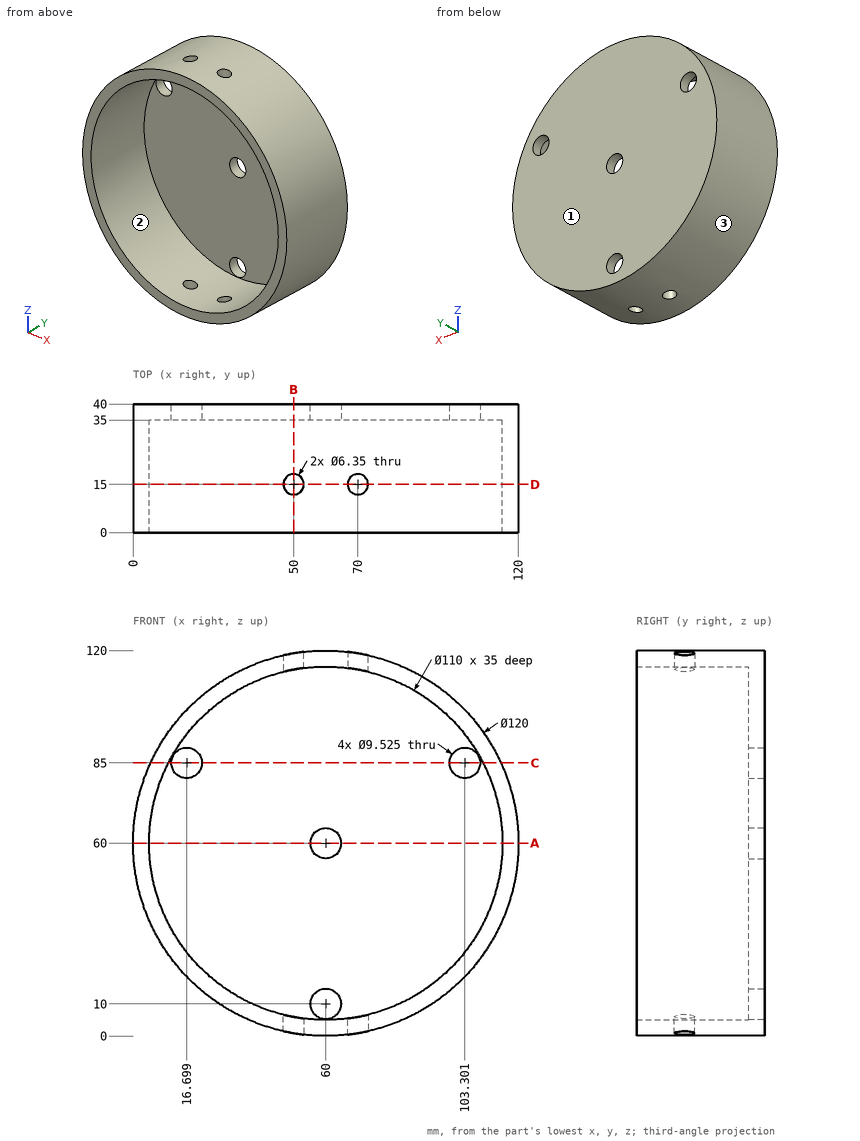
Study the drawing (mm; zero at the part's minimum x, y, z) and answer. Give positions to 0.01 mm unless a question says otherwise; leave off trailing zeros. Loops run counter-clockwise (first coordinate to the right, second up) from the corner with the lowest first, then second, coordinate; pieces in that order, holes last. Notation, with made-up numbers: (84.5, -19) -> (94.5, -19) arc R31 ccw to (94.5, 6) -> close; hole circle Ø7 at (88, -6.75). An arc over 180 degrees is marked (long way). Write item = value, one per line. Start each with the question number.
(1) Find section D-D on y = 15. Give the vertices of the cut face in (x, z) (1 decimal), and give its area (3 significant figures).
(2) The mould has two halves that part along Z. Classify the marked faces 1, 2 and 3: +Z half, -Z half, draft (parallel to the pull), parting line (faces both ways), or undercut.
(3) Given pin 1 Ø4 at (y, z) = (27, 72.5) entering from +X; pin 2 Ø4 at (y, z) = (25, 58) entering from -X; pin 3 Ø8.5 at (x, y) = (50, 15) entering from -Z; pin 4 Ø2 at (x, y) = (51.5, 29) entering from -Z, each flat-ended and moving along its own axis, determine where each tip first touches the part or whether it passes through.
(4) Find section A-A on z = 60. Give the vertices of the cut face in (x, y).
(5) Find section B-B on x = 50. Give the vertices of the cut face in (y, z) (1 decimal).
(6) Find the intervals of material crossed by probe 1 along Z at (x, y) = (60, 36); probe 2 along Z at (x, y) = (60.5, 16); probe 3 along Y at (x, z) = (50, 115.75) (1 decimal), in increasing order. Write a range as from..to.
(7) Find section C-C on z = 85. Give the vertices of the cut face in (x, y).
From the geometry:
q1.outline = (46.8, 1.5) -> (46.8, 6.6) arc R55 cw to (46.8, 113.4) -> (46.8, 118.5) arc R60 ccw to start; (53.2, 0.4) arc R60 ccw to (66.8, 0.4) -> (66.8, 5.4) arc R55 cw to (53.2, 5.4) -> close; (53.2, 114.6) arc R55 cw to (66.8, 114.6) -> (66.8, 119.6) arc R60 ccw to (53.2, 119.6) -> close; (73.2, 1.5) arc R60 ccw to (73.2, 118.5) -> (73.2, 113.4) arc R55 cw to (73.2, 6.6) -> close
q1.area = 1,680 mm^2
q2.face_1 = draft
q2.face_2 = undercut
q2.face_3 = parting line
q3.pin_1 = 119.07
q3.pin_2 = 0
q3.pin_3 = 0.28
q3.pin_4 = 0.47
q4.outline = (0, 0) -> (5, 0) -> (5, 35) -> (55.24, 35) -> (55.24, 40) -> (0, 40) -> close; (64.76, 35) -> (115, 35) -> (115, 0) -> (120, 0) -> (120, 40) -> (64.76, 40) -> close
q5.outline = (0, 0.8) -> (11.8, 0.8) -> (11.8, 5.9) -> (0, 5.9) -> close; (0, 114.1) -> (11.8, 114.1) -> (11.8, 119.2) -> (0, 119.2) -> close; (18.2, 0.8) -> (40, 0.8) -> (40, 119.2) -> (18.2, 119.2) -> (18.2, 114.1) -> (35, 114.1) -> (35, 5.9) -> (18.2, 5.9) -> close
q6.probe_1 = 0..5.24, 14.76..55.24, 64.76..120
q6.probe_2 = 0..5, 115..120
q6.probe_3 = 0..11.8, 18.2..40
q7.outline = (5.46, 0) -> (11.01, 0) -> (11.01, 35) -> (11.94, 35) -> (11.94, 40) -> (5.46, 40) -> close; (21.46, 35) -> (98.54, 35) -> (98.54, 40) -> (21.46, 40) -> close; (108.06, 35) -> (108.99, 35) -> (108.99, 0) -> (114.54, 0) -> (114.54, 40) -> (108.06, 40) -> close
